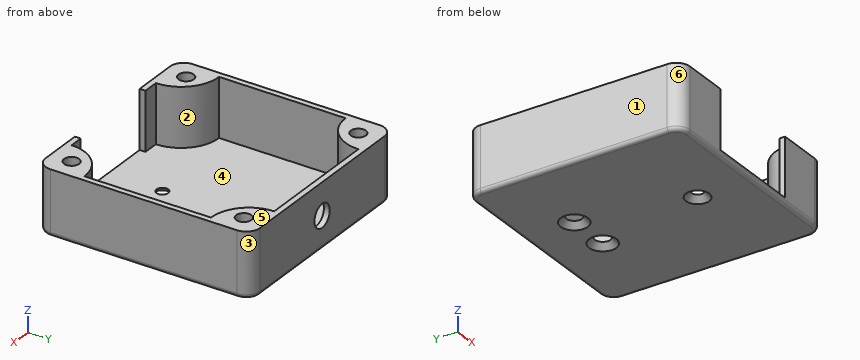
from build123d import *

# Parameters (mm, degrees)
PAD_DEPTH               = 16.5
POCKET_DEPTH            = 15
SKETCH002_R             = 1.95
PAD001_DEPTH            = 15
SKETCH002_MIRRORED_2_R  = 1.95
PAD001_MIRRORED_2_DEPTH = 15
FILLET_R                = 1
SKETCH008_W             = 25
SKETCH008_H             = 15
POCKET003_DEPTH         = 5
SKETCH010_R             = 1.5
SKETCH010_R_2           = 2
POCKET004_DEPTH         = 5
SKETCH011_R             = 2.95
POCKET005_DEPTH         = 5
CHAMFER_SIZE            = 1.499


with BuildPart() as part:
    # Sketch → Pad (new body)
    with BuildSketch(Plane.XY):
        with BuildLine():
            Line((-24, 27.5), (24, 27.5))
            ThreePointArc((27.5, 24), (26.474874, 26.474874), (24, 27.5))
            Line((27.5, 24), (27.5, -24))
            ThreePointArc((24, -27.5), (26.474874, -26.474874), (27.5, -24))
            Line((24, -27.5), (-24, -27.5))
            ThreePointArc((-27.5, -24), (-26.474874, -26.474874), (-24, -27.5))
            Line((-27.5, -24), (-27.5, 24))
            ThreePointArc((-24, 27.5), (-26.474874, 26.474874), (-27.5, 24))
        make_face()
    extrude(amount=PAD_DEPTH)

    # Sketch001 (on Face10 of Pad) → Pocket (cut)
    with BuildSketch(Plane.XY.offset(16.5)):
        with BuildLine():
            Line((-24.25, 26), (24.25, 26))
            ThreePointArc((26, 24.25), (25.487437, 25.487437), (24.25, 26))
            Line((26, 24.25), (26, -24.25))
            ThreePointArc((24.25, -26), (25.487437, -25.487437), (26, -24.25))
            Line((24.25, -26), (-24.25, -26))
            ThreePointArc((-26, -24.25), (-25.487437, -25.487437), (-24.25, -26))
            Line((-26, -24.25), (-26, 24.25))
            ThreePointArc((-24.25, 26), (-25.487437, 25.487437), (-26, 24.25))
        make_face()
    extrude(amount=-POCKET_DEPTH, mode=Mode.SUBTRACT)

    # Sketch002 (on Face19 of Pocket) → Pad001 (join)
    with BuildSketch(Plane.XY.offset(1.5)):
        with BuildLine():
            Line((-26, 16.25), (-26, 26))
            Line((-26, 26), (-16.25, 26))
            ThreePointArc((-26, 16.25), (-19.105709, 19.105709), (-16.25, 26))
        make_face()
        with Locations((-22.1, 22.1)):
            Circle(SKETCH002_R, mode=Mode.SUBTRACT)
    pad001 = extrude(amount=PAD001_DEPTH)

    # Sketch002 Mirrored 2 → Pad001 Mirrored 2 (add)
    with BuildSketch(Plane(origin=(0, 0, 1.5), x_dir=(-1, 0, 0), z_dir=(0, 0, -1))):
        with BuildLine():
            Line((-26, 16.25), (-26, 26))
            Line((-26, 26), (-16.25, 26))
            ThreePointArc((-26, 16.25), (-19.105709, 19.105709), (-16.25, 26))
        make_face()
        with Locations((-22.1, 22.1)):
            Circle(SKETCH002_MIRRORED_2_R, mode=Mode.SUBTRACT)
    pad001_mirrored_2 = extrude(amount=-PAD001_MIRRORED_2_DEPTH)

    # Mirrored001: Pad001, Pad001 Mirrored 2 across Sketch002 H_Axis
    add(pad001.mirror(Plane(origin=(0, 0, 1.5), x_dir=(0, 0, 1), z_dir=(0, 1, 0))))
    add(pad001_mirrored_2.mirror(Plane(origin=(0, 0, 1.5), x_dir=(0, 0, 1), z_dir=(0, 1, 0))))

    # Fillet
    fillet_edges = [part.edges().sort_by_distance(p)[0] for p in [
        (-27.5, 0, 0),
        (-26.474874, 26.474874, 0),
        (0, 27.5, 0),
        (26.474874, 26.474874, 0),
        (27.5, 0, 0),
        (26.474874, -26.474874, 0),
        (0, -27.5, 0),
        (-26.474874, -26.474874, 0),
    ]]
    fillet(fillet_edges, radius=FILLET_R)

    # Sketch008 (on Face7 of Fillet) → Pocket003 (cut)
    with BuildSketch(Plane.XZ.offset(27.5)):
        with Locations((0.25, 9)):
            Rectangle(SKETCH008_W, SKETCH008_H)
    extrude(amount=-POCKET003_DEPTH, mode=Mode.SUBTRACT)

    # Sketch010 (on Face35 of Pocket003) → Pocket004 (cut)
    with BuildSketch(Plane.XY.offset(1.5)):
        with Locations((0, -13.5)):
            Circle(SKETCH010_R)
        with Locations((-5.5, 14.5)):
            Circle(SKETCH010_R_2)
        with Locations((5.5, 14.5)):
            Circle(SKETCH010_R_2)
    extrude(amount=-POCKET004_DEPTH, mode=Mode.SUBTRACT)

    # Sketch011 (on Face10 of Pocket004) → Pocket005 (cut)
    with BuildSketch(Plane(origin=(0, 27.5, 0), x_dir=(-1, 0, 0), z_dir=(0, 1, 0))):
        with Locations((0, 8.25)):
            Circle(SKETCH011_R)
    extrude(amount=-POCKET005_DEPTH, mode=Mode.SUBTRACT)

    # Chamfer
    chamfer_edges = [part.edges().sort_by_distance(p)[0] for p in [
        (3.5, 14.5, 0),
        (-7.5, 14.5, 0),
        (-1.5, -13.5, 0),
    ]]
    chamfer(chamfer_edges, length=CHAMFER_SIZE)


solid = part.part
For this review, take the finished solid that the model builds, in its own axes (mm). Face numbers are marked on the shaded views. A direction names the side the tool comes from. Give positions to 0.01 mm unless a question says otherwise; leave off trailing zeros. Loops run counter-clockwise (first coordinate to the right, second up) from the corner with the lowest first, then second, coordinate; pieces in that order, holes last. Notation, with made-up numbers: M 89,85.5 L 134,85.5 A24 cw 134,108.5 Z; hole C 44.5,-27 d3. An arc over 180 degrees is marked long. Put each result on its own line as item: value. Start each with the question number.
(1) Add section B-B, the plane y = -5.5. Write out the cut boundary in (x, z), then the cut area to 3 significant figures.
(2) Wall thickness on L1, parallel to X at y = 15.5, z = 4; L2, parallel to X at y = -22.1, z = 8: over which ranges is each line inside the solid? List them lowest first.
(3) The part is to be moulded in two halves that separate along Y. For the marked faces 3, 4, 5 and 6, say which applies: +Y half, -Y half, draft (parallel to the pull), parting line (faces both ways), or undercut.
(4) Machinability: for the marked faces 1 and 2, which of the approach directions +Z, -Z, +X, -X, +Y, -Y give a long, thin tool a straight path to every point of the face, cutting with its end or side? Answer none if there is none.
(5) For pin 1 (1.2 mm diameter, centred on x = 22.5, y = 21.5, fed in from +Z), flat-tipped, find the tip position at first contact; note if it passes through.
(6) Add section D-D, the plane z = 4. Write out the cut boundary in (x, y).
(7) Add section C-C, the plane z = 10. Write out the cut boundary in (x, y).
Result:
1. outline: M -27.5,1 A1 ccw -26.5,0 L 26.5,0 A1 ccw 27.5,1 L 27.5,16.5 L 26,16.5 L 26,1.5 L -26,1.5 L -26,16.5 L -27.5,16.5 Z
1. area: 127 mm^2
2. L1: x = -27.5 to -26, 26 to 27.5
2. L2: x = -27.5 to -24.05, -20.15 to -17.06, 17.06 to 20.15, 24.05 to 27.5
3. face 3: +Y half
3. face 4: undercut
3. face 5: draft
3. face 6: -Y half
4. face 1: +Z, -Z, -X, +Y, -Y
4. face 2: +Z
5. pin 1: stops at z = 1.5
6. outline: M -27.5,-24 A3.5 ccw -24,-27.5 L -12.25,-27.5 L -12.25,-26 L -16.25,-26 A9.75 ccw -26,-16.25 L -26,16.25 A9.75 ccw -16.25,26 L 16.25,26 A9.75 ccw 26,16.25 L 26,-16.25 A9.75 ccw 16.25,-26 L 12.75,-26 L 12.75,-27.5 L 24,-27.5 A3.5 ccw 27.5,-24 L 27.5,24 A3.5 ccw 24,27.5 L -24,27.5 A3.5 ccw -27.5,24 Z; hole C -22.1,-22.1 d3.9; hole C -22.1,22.1 d3.9; hole C 22.1,-22.1 d3.9; hole C 22.1,22.1 d3.9
7. outline: M -27.5,-24 A3.5 ccw -24,-27.5 L -12.25,-27.5 L -12.25,-26 L -16.25,-26 A9.75 ccw -26,-16.25 L -26,16.25 A9.75 ccw -16.25,26 L -2.37,26 L -2.37,27.5 L -24,27.5 A3.5 ccw -27.5,24 Z; M 2.37,26 L 16.25,26 A9.75 ccw 26,16.25 L 26,-16.25 A9.75 ccw 16.25,-26 L 12.75,-26 L 12.75,-27.5 L 24,-27.5 A3.5 ccw 27.5,-24 L 27.5,24 A3.5 ccw 24,27.5 L 2.37,27.5 Z; hole C -22.1,-22.1 d3.9; hole C -22.1,22.1 d3.9; hole C 22.1,-22.1 d3.9; hole C 22.1,22.1 d3.9
